Read the model definition and answer for the solid it produces. Units are mm, in the model's axes. Coordinates: 2 decimals unless noted, no trailing zeros. Order: outer loops, then holes, each group sorted by start corner. A loop starts at its lowest first (then second) coordinate and runs counter-clockwise, first axis right, second up. Notation, with made-up numbers: M -38.75,1 L -15.75,1 A16 cw -15.75,5 Z; hole C 51,21.25 d4. An arc over 180 degrees is marked long. Put each result on its own line as item: value.
from build123d import *

# Parameters (mm, degrees)
SKETCH1_R                                       = 10
SKETCH1_R_2                                     = 3
BOSS_EXTRUDE1_DEPTH                             = 2.5
CSK_FOR_M2_FLAT_HEAD_MACHINE_SCREW3_D           = 2.2
CSK_FOR_M2_FLAT_HEAD_MACHINE_SCREW3_CSINK_D     = 4.4
CSK_FOR_M2_FLAT_HEAD_MACHINE_SCREW3_CSINK_ANGLE = 90


with BuildPart() as part:
    # Sketch1 → Boss-Extrude1 (new body)
    # profile 1 of 2: a face of its own
    with BuildSketch(Plane.XY):
        Circle(SKETCH1_R)
        Polygon((4.996174644, 1.623355548), (0, 5.253288904), (-4.996174644, 1.623355548), (-3.087805744, -4.25), (3.087805744, -4.25), align=None, mode=Mode.SUBTRACT)
    # profile 2 of 2: a face of its own
    with BuildSketch(Plane.XY):
        Polygon((3.087805744, -4.25), (4.996174644, 1.623355548), (0, 5.253288904), (-4.996174644, 1.623355548), (-3.087805744, -4.25), align=None)
        Circle(SKETCH1_R_2, mode=Mode.SUBTRACT)
    extrude(amount=BOSS_EXTRUDE1_DEPTH)

    # CSK for M2 Flat Head Machine Screw3 (through all)
    with Locations(Plane.XY.offset(2.5)):
        with Locations((0, 5.253288904), (4.996174644, 1.623355548), (3.087805744, -4.25), (-4.996174644, 1.623355548), (-3.087805744, -4.25)):
            CounterSinkHole(CSK_FOR_M2_FLAT_HEAD_MACHINE_SCREW3_D / 2, CSK_FOR_M2_FLAT_HEAD_MACHINE_SCREW3_CSINK_D / 2, counter_sink_angle=CSK_FOR_M2_FLAT_HEAD_MACHINE_SCREW3_CSINK_ANGLE)


solid = part.part
Q1. Find section B-B on y = -4.25. Write down the section's boundary in (x, z).
Answers below:
outline: M -9.05,0 L -4.19,0 L -4.19,1.4 L -5.29,2.5 L -9.05,2.5 Z; M -1.99,0 L 1.99,0 L 1.99,1.4 L 0.89,2.5 L -0.89,2.5 L -1.99,1.4 Z; M 4.19,0 L 9.05,0 L 9.05,2.5 L 5.29,2.5 L 4.19,1.4 Z
Q2. Given pin 1 (3.5 mm diameter, centred on x = 0, y = 0, fed in from -Z); pin 2 (3.5 mm diameter, centred on x = 3.09, y = -4.25, fed in from +Z); pin 3 (1.5 mm diameter, centred on y = -4, z = 1, fed in from +X); pin 4 (1.5 mm diameter, centred on y = 1.5, z = 1, fed in from +X), each flat-ended and moving along its own axis, determine where each tip first touches the part or whether it passes through.
Answers below:
pin 1: passes through
pin 2: stops at z = 2.05
pin 3: stops at x = 9.46
pin 4: stops at x = 9.97
Q3. For a pull along X with two mould halves and no side action, classify faces 1 (the face through (-3.9, 1.7, 0.7)), 2 (the face through (2.1, 2.4, 0)), 3 (the face through (-2.17, -9.76, 1.23)) as +X half, -X half, draft (parallel to the pull), parting line (faces both ways), or undercut.
Answers below:
face 1: undercut
face 2: draft
face 3: parting line
Q4. Find section A-A on x = 0. Write down the section's boundary in (y, z), plus the area to 3 significant figures.
Answers below:
outline: M -10,0 L -3,0 L -3,2.5 L -10,2.5 Z; M 3,0 L 4.15,0 L 4.15,1.4 L 3.05,2.5 L 3,2.5 Z; M 6.35,0 L 10,0 L 10,2.5 L 7.45,2.5 L 6.35,1.4 Z
area: 28.3 mm^2
Q5. Find section D-D on z = 1.8. Write down the section's boundary in (x, y).
Answers below:
outline: C 0,0 d20; hole C -5,1.62 d3; hole C -3.09,-4.25 d3; hole C 0,0 d6; hole C 0,5.25 d3; hole C 3.09,-4.25 d3; hole C 5,1.62 d3
Q6. Find section C-C on z = 0.4. Write down the section's boundary in (x, y).
Answers below:
outline: C 0,0 d20; hole C -5,1.62 d2.2; hole C -3.09,-4.25 d2.2; hole C 0,0 d6; hole C 0,5.25 d2.2; hole C 3.09,-4.25 d2.2; hole C 5,1.62 d2.2
Q7. Consider line 1 along X through (y, z) = (-4.25, 0.5); line 2 along Y through (x, z) = (2.75, 1.9); line 3 along Y through (x, z) = (0.25, 0.9). Determine where each line is inside the solid, lowest interval first.
Answers below:
line 1: x = -9.05 to -4.19, -1.99 to 1.99, 4.19 to 9.05
line 2: y = -9.61 to -5.81, -2.69 to -1.2, 1.2 to 9.61
line 3: y = -10 to -2.99, 2.99 to 4.18, 6.32 to 10
